Job drawing, mm, ordinate dimensions from the low corner. One solid piece. Coordinates: 2 decimals unless noted, no trailing zeros. Loops run counter-clockwise (first coordinate to the right, second up) from the corner with the lowest first, then second, coordinate; pieces in that order, holes last. Notation, with made-up numbers: (46.5, 13.5) -> (82.5, 13.5) arc R17 ccw to (82.5, 40.5) -> close; hole circle Ø4 at (26, -29). An arc over 180 degrees is marked (long way). Answer as CSV lines item,"result". Start each with the question number.
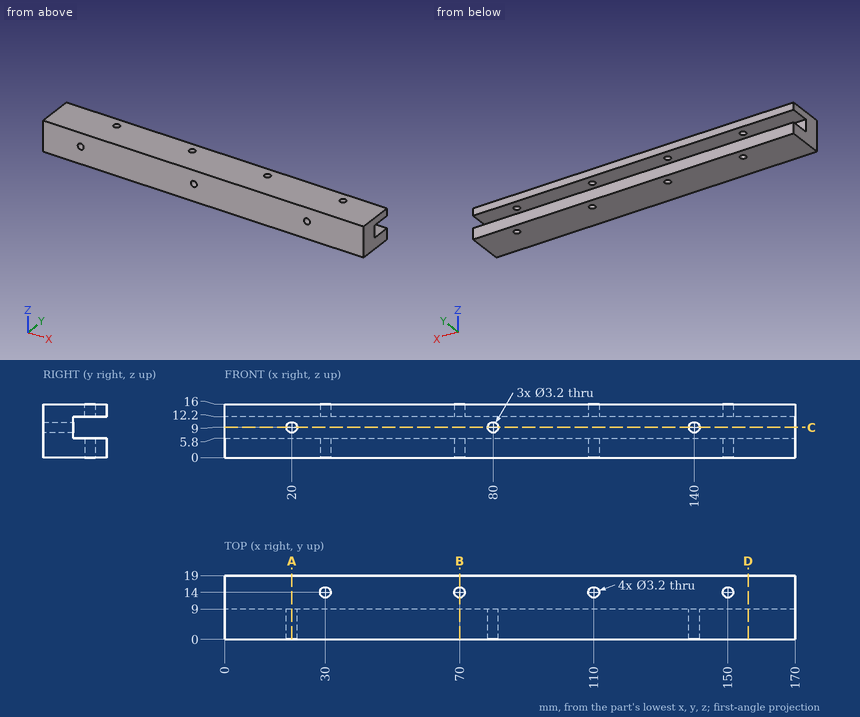
Item 1: Flat gauge pins, fed straight in: pin 1 Ø3 at (x, y) = (81.5, 14) entering from -Z; pin 2 Ø3.5 at (x, z) = (80, 9) entering from +Y; pin 3 Ø2.5 at (x, y) = (70, 14) entering from -Z. Where does each tip first touch, or does it go through?
Item 2: Saw through at B-B (x = 70). Write the cut outline in (y, z).
Item 3: Saw through at A-A (x = 20). Write the cut outline in (y, z).
Item 4: Saw through at C-C (z = 9). Write the cut outline in (x, y), plus the area to 3 significant figures.
Item 5: Wall check: probe 1 along X at (y, z) = (14, 2.8); probe 2 along Z at (x, y) = (20, 6); probe 3 along Z at (x, y) = (147.5, 16.5). Give the ranges that are in metal, low to high.
Item 6: Saw through at D-D (x = 156). Write the cut outline in (y, z), plus the area to 3 significant figures.
Geometry check:
1,pin 1,"z = 0"
1,pin 2,"y = 9"
1,pin 3,"through"
2,outline,"(0, 0) -> (12.4, 0) -> (12.4, 5.8) -> (9, 5.8) -> (9, 12.2) -> (12.4, 12.2) -> (12.4, 16) -> (0, 16) -> close; (15.6, 0) -> (19, 0) -> (19, 5.8) -> (15.6, 5.8) -> close; (15.6, 12.2) -> (19, 12.2) -> (19, 16) -> (15.6, 16) -> close"
3,outline,"(0, 0) -> (19, 0) -> (19, 5.8) -> (9, 5.8) -> (9, 7.4) -> (0, 7.4) -> close; (0, 10.6) -> (9, 10.6) -> (9, 12.2) -> (19, 12.2) -> (19, 16) -> (0, 16) -> close"
4,outline,"(0, 0) -> (18.4, 0) -> (18.4, 9) -> (0, 9) -> close; (21.6, 0) -> (78.4, 0) -> (78.4, 9) -> (21.6, 9) -> close; (81.6, 0) -> (138.4, 0) -> (138.4, 9) -> (81.6, 9) -> close; (141.6, 0) -> (170, 0) -> (170, 9) -> (141.6, 9) -> close"
4,area,"1,440 mm2"
5,probe 1,"0 to 28.4, 31.6 to 68.4, 71.6 to 108.4, 111.6 to 148.4, 151.6 to 170"
5,probe 2,"0 to 7.4, 10.6 to 16"
5,probe 3,"0 to 5.8, 12.2 to 16"
6,outline,"(0, 0) -> (19, 0) -> (19, 5.8) -> (9, 5.8) -> (9, 12.2) -> (19, 12.2) -> (19, 16) -> (0, 16) -> close"
6,area,"240 mm2"
